Build history of the part. All positions in model axes, mm. Give positions to 0.01 mm unless a question says otherwise; leave off trailing zeros. Write each loop counter-clockwise with the first axis right and the second up, starting at its lowest first coordinate (ties: lowest second). Pieces come first, ordered by that corner, then holes. Notation, with made-up numbers: M 47,54 L 97,54 A15 ccw 97,68 Z; hole C 69.5,18 d5. An arc over 180 degrees is marked long. Return JSON: item names as keys, results as strings. Group by question number.
Q1. Flat gauge pins, fed straight in: pin 1 Ø6.5 at (x, y) = (16.25, -15) entering from -Z; pin 2 Ø1 at (y, z) = (-13, -3) entering from -X; pin 3 Ø4.5 at (x, z) = (47, -7) entering from +Y. Where does each tip first touch, or does it go through?
Q2. Band-saw the part on C-C, the plane x = 111.75. Give the cut face in (y, z), then the cut area to 3 significant figures.
Q3. Band-saw the part on A-A, the plane x = -54. Give the cut face in (y, z).
Q4. Wall check: probe 1 along Y at (x, z) = (77.75, 1); probe 2 along X at (y, z) = (11, 2.25); probe 3 along Y at (x, z) = (-43.75, 1.95). Give the ranges that are in metal, low to high.
Q5. Band-saw the part on B-B, the plane y = 24.5. Give the cut face in (x, z), then the cut area to 3 significant figures.
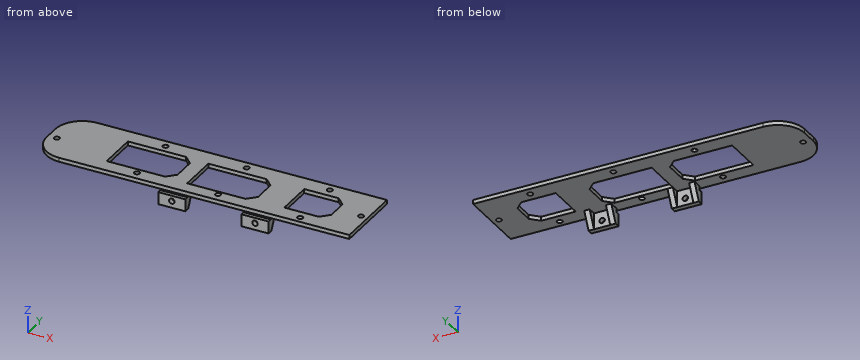
from build123d import *

# Parameters (mm, degrees)
SKETCH1_W            = 229.5
SKETCH1_H            = 49
BOSS_EXTRUDE1_DEPTH  = 3
SKETCH3_W            = 229.5
SKETCH3_H            = 3
BOSS_EXTRUDE2_DEPTH  = 6
SKETCH2_R            = 2
CUT_EXTRUDE1_DEPTH   = 31.956
SKETCH4_R            = 2
CUT_EXTRUDE2_DEPTH   = 31.956
BOSS_EXTRUDE3_DEPTH  = 3
SKETCH10_W           = 229.5
SKETCH10_H           = 2.9625
CUT_EXTRUDE5_DEPTH   = 11.382
BOSS_EXTRUDE4_DEPTH  = 12
SKETCH13_R           = 2
CUT_EXTRUDE7_DEPTH   = 15
BOSS_EXTRUDE5_DEPTH  = 4
BOSS_EXTRUDE6_DEPTH  = 4
BOSS_EXTRUDE7_DEPTH  = 4
BOSS_EXTRUDE8_DEPTH  = 4
SKETCH19_W           = 3
SKETCH19_H           = 52.0375
BOSS_EXTRUDE9_DEPTH  = 2.984
CUT_EXTRUDE8_DEPTH   = 20.764
SKETCH23_W           = 3
SKETCH23_H           = 52.0375
BOSS_EXTRUDE10_DEPTH = 2
SKETCH24_W           = 20
SKETCH24_H           = 3
CUT_EXTRUDE9_DEPTH   = 3


with BuildPart() as part:
    # Sketch1 → Boss-Extrude1 (new body)
    with BuildSketch(Plane.XY):
        Rectangle(SKETCH1_W, SKETCH1_H)
    extrude(amount=BOSS_EXTRUDE1_DEPTH)

    # Sketch3 → Boss-Extrude2 (add)
    with BuildSketch(Plane(origin=(0, 24.5, 0), x_dir=(1, 0, 0), z_dir=(0, 1, 0))):
        with Locations((0, -1.5)):
            Rectangle(SKETCH3_W, SKETCH3_H)
    extrude(amount=BOSS_EXTRUDE2_DEPTH)

    # Sketch2 → Cut-Extrude1 (cut)
    with BuildSketch(Plane.XY.offset(3)):
        with Locations((111.75, 4)):
            Circle(SKETCH2_R)
        with Locations((-111.25, 0.5)):
            Circle(SKETCH2_R)
        with Locations((-43.75, 24.5)):
            Circle(SKETCH2_R)
        with Locations((16.25, 24.5)):
            Circle(SKETCH2_R)
        with Locations((77.75, 24.5)):
            Circle(SKETCH2_R)
    extrude(amount=-CUT_EXTRUDE1_DEPTH, mode=Mode.SUBTRACT)

    # Sketch4 → Cut-Extrude2 (cut)
    with BuildSketch(Plane.XY.offset(3)):
        Polygon((87.924883288, 17.681445753), (62.424883288, 17.681445753), (62.424883288, -9.818554247), (87.924883288, -9.818554247), (93.924883288, -3.818554247), (93.924883288, 11.681445753), align=None)
        Polygon((-19.25, -4.71), (-19.25, 12.5), (-25.25, 18.5), (-68.43, 18.5), (-68.43, -10.71), (-25.25, -10.71), align=None)
        Polygon((-8.429595307, -11.664), (34.750404693, -11.664), (40.750404693, -5.664), (40.750404693, 11.546), (34.750404693, 17.546), (-8.429595307, 17.546), align=None)
        with Locations((-43.75, -15)):
            Circle(SKETCH4_R)
        with Locations((16.25, -15)):
            Circle(SKETCH4_R)
        with Locations((77.75, -16.5)):
            Circle(SKETCH4_R)
    extrude(amount=-CUT_EXTRUDE2_DEPTH, mode=Mode.SUBTRACT)

    # Sketch5 → Boss-Extrude3 (add)
    with BuildSketch(Plane.XY.offset(3)):
        with BuildLine():
            ThreePointArc((-114.75, 5.373397172), (-117.25, 0.5), (-114.75, -4.373397172))
            Line((-114.75, -4.373397172), (-114.75, 5.373397172))
        make_face()
    extrude(amount=-BOSS_EXTRUDE3_DEPTH)

    # Sketch10 → Cut-Extrude5 (cut)
    with BuildSketch(Plane(origin=(0, 0, 0), x_dir=(-1, 0, 0), z_dir=(0, 0, -1))):
        with Locations((0, -23.01875)):
            Rectangle(SKETCH10_W, SKETCH10_H)
    extrude(amount=-CUT_EXTRUDE5_DEPTH, mode=Mode.SUBTRACT)

    # Sketch12 → Boss-Extrude4 (add)
    with BuildSketch(Plane(origin=(0, 0, 0), x_dir=(-1, 0, 0), z_dir=(0, 0, -1))):
        Polygon((-47, -21.5375), (-41, -21.5375), (-41, -17.5375), (-53, -17.5375), (-53, -21.5375), align=None)
        Polygon((8.5, -21.5375), (13.75, -21.5375), (20.5, -21.5375), (20.5, -17.5375), (8.5, -17.5375), align=None)
    extrude(amount=BOSS_EXTRUDE4_DEPTH)

    # Sketch13 → Cut-Extrude7 (cut)
    with BuildSketch(Plane(origin=(0, -17.5375, 0), x_dir=(1, 0, 0), z_dir=(0, 1, 0))):
        with Locations(Location((-14.5, 7, 0), (0, 0, 270))):
            Circle(SKETCH13_R)
        with Locations(Location((47, 7, 0), (0, 0, 270))):
            Circle(SKETCH13_R)
    extrude(amount=-CUT_EXTRUDE7_DEPTH, mode=Mode.SUBTRACT)

    # Sketch14 → Boss-Extrude5 (add)
    with BuildSketch(Plane(origin=(53, 0, 0), x_dir=(0, 0, -1), z_dir=(1, 0, 0))):
        Polygon((0, -17.5375), (0, -11.5375), (12, -17.5375), (12, -21.5375), (0, -21.5375), align=None)
    extrude(amount=BOSS_EXTRUDE5_DEPTH)

    # Sketch15 → Boss-Extrude6 (add)
    with BuildSketch(Plane.ZY.offset(-41)):
        Polygon((0, -17.5375), (0, -11.5375), (-12, -17.5375), (-12, -21.5375), (0, -21.5375), align=None)
    extrude(amount=BOSS_EXTRUDE6_DEPTH)

    # Sketch16 → Boss-Extrude7 (add)
    with BuildSketch(Plane(origin=(-8.5, 0, 0), x_dir=(0, 0, -1), z_dir=(1, 0, 0))):
        Polygon((0, -17.5375), (0, -11.5375), (12, -17.5375), (12, -21.5375), (0, -21.5375), align=None)
    extrude(amount=BOSS_EXTRUDE7_DEPTH)

    # Sketch17 → Boss-Extrude8 (add)
    with BuildSketch(Plane.ZY.offset(20.5)):
        Polygon((0, -17.5375), (0, -11.5375), (-12, -17.5375), (-12, -21.5375), (0, -21.5375), align=None)
    extrude(amount=BOSS_EXTRUDE8_DEPTH)

    # Sketch19 → Boss-Extrude9 (add)
    with BuildSketch(Plane.ZY.offset(114.75)):
        with Locations((1.5, 4.48125)):
            Rectangle(SKETCH19_W, SKETCH19_H)
    extrude(amount=BOSS_EXTRUDE9_DEPTH)

    # Sketch20 → Cut-Extrude8 (cut)
    with BuildSketch(Plane.XY.offset(3)):
        with BuildLine():
            ThreePointArc((-117.734, 10.5), (-111.876135624, 24.642135624), (-97.734, 30.5))
            Line((-97.734, 30.5), (-117.734, 30.5))
            Line((-117.734, 30.5), (-117.734, 10.5))
        make_face()
        with BuildLine():
            ThreePointArc((-97.734, -21.5375), (-111.876135624, -15.679635624), (-117.734, -1.5375))
            Line((-117.734, -1.5375), (-117.734, -21.5375))
            Line((-117.734, -21.5375), (-97.734, -21.5375))
        make_face()
    extrude(amount=-CUT_EXTRUDE8_DEPTH, mode=Mode.SUBTRACT)

    # Sketch23 → Boss-Extrude10 (add)
    with BuildSketch(Plane(origin=(114.75, 0, 0), x_dir=(0, 0, -1), z_dir=(1, 0, 0))):
        with Locations((-1.5, 4.48125)):
            Rectangle(SKETCH23_W, SKETCH23_H)
    extrude(amount=BOSS_EXTRUDE10_DEPTH)

    # Sketch24 → Cut-Extrude9 (cut)
    with BuildSketch(Plane.XZ.offset(21.5375)):
        with Locations((-14.5, -1.5)):
            Rectangle(SKETCH24_W, SKETCH24_H)
        with Locations((47, -1.5)):
            Rectangle(SKETCH24_W, SKETCH24_H)
    extrude(amount=-CUT_EXTRUDE9_DEPTH, mode=Mode.SUBTRACT)


solid = part.part
From the geometry:
{
 "1": {"pin 1": "stops at z = 0", "pin 2": "stops at x = -24.5", "pin 3": "stops at y = -17.54"},
 "2": {"outline": "M -21.54,0 L 2,0 L 2,3 L -21.54,3 Z; M 6,0 L 30.5,0 L 30.5,3 L 6,3 Z", "area": "144 mm^2"},
 "3": {"outline": "M -21.54,0 L -10.71,0 L -10.71,3 L -21.54,3 Z; M 18.5,0 L 30.5,0 L 30.5,3 L 18.5,3 Z"},
 "4": {"probe 1": "y = -21.54 to -18.5, -14.5 to -9.82, 17.68 to 22.5, 26.5 to 30.5", "probe 2": "x = -117.73 to -68.43, -19.25 to -8.43, 40.75 to 62.42, 93.92 to 116.75", "probe 3": "y = -21.54 to -17, -13 to -10.71, 18.5 to 22.5, 26.5 to 30.5"},
 "5": {"outline": "M -112.02,0 L -45.75,0 L -45.75,3 L -112.02,3 Z; M -41.75,0 L 14.25,0 L 14.25,3 L -41.75,3 Z; M 18.25,0 L 75.75,0 L 75.75,3 L 18.25,3 Z; M 79.75,0 L 116.75,0 L 116.75,3 L 79.75,3 Z", "area": "650 mm^2"}
}
